```python
from build123d import *

# Parameters (mm, degrees)
SKETCH_3_R      = 2.25
EXTRUDE_1_DEPTH = 11
SKETCH_4_R      = 0.4
FILLET_1_R      = 0.5


with BuildPart() as part:
    # Эскиз3 → Вытянуть1 (new body)
    with BuildSketch(Plane(origin=(2.5, 0, 0), x_dir=(0, 0, -1), z_dir=(1, 0, 0))):
        with Locations((-2.25, 0)):
            Circle(SKETCH_3_R)
    extrude(amount=EXTRUDE_1_DEPTH)

    # По траектории1: sweep along a path in Эскиз5
    with BuildLine(Plane(origin=(0, 0, 0), x_dir=(1, 0, 0), z_dir=(0, 1, 0))) as sweep_1_path:
        Line((0, 5.25), (0, -0.25))
        ThreePointArc((0, -0.25), (0.585786438, -1.664213562), (2, -2.25))
        Line((2, -2.25), (2.965757317, -2.25))
        Line((2.965757317, -2.25), (14, -2.25))
        ThreePointArc((14, -2.25), (15.414213562, -1.664213562), (16, -0.25))
        Line((16, -0.25), (16, 5.25))
    # Эскиз4 → По траектории1 (sweep)
    with BuildSketch(Plane.XY.offset(-5.25)):
        Circle(SKETCH_4_R)
    sweep(path=sweep_1_path.line)

    # Скругление1
    fillet_1_edges = [part.edges().sort_by_distance(p)[0] for p in [
        (2.5, 0, 4.5),
        (13.5, 0, 4.5),
    ]]
    fillet(fillet_1_edges, radius=FILLET_1_R)


solid = part.part
```
The listing builds one solid part. Answer for the finished solid, in the listing's coordinates (mm). Give positions to 0.01 mm unless a question says otherwise; leave off trailing zeros. Order: outer loops, then holes, each group sorted by start corner. A loop starts at its lowest first (then second) coordinate and runs counter-clockwise, first axis right, second up.
1) Find section A-A on y = 0. Write down the section's boundary in (x, z).
Reported:
outline: (-0.4, -5.25) - (0.4, -5.25) - (0.4, 0.25) arc R1.6 cw to (2, 1.85) - (2.5, 1.85) - (2.5, 0.5) arc R0.5 ccw to (3, 0) - (13, 0) arc R0.5 ccw to (13.5, 0.5) - (13.5, 1.85) - (14, 1.85) arc R1.6 cw to (15.6, 0.25) - (15.6, -5.25) - (16.4, -5.25) - (16.4, 0.25) arc R2.4 ccw to (14, 2.65) - (13.5, 2.65) - (13.5, 4) arc R0.5 ccw to (13, 4.5) - (3, 4.5) arc R0.5 ccw to (2.5, 4) - (2.5, 2.65) - (2, 2.65) arc R2.4 ccw to (-0.4, 0.25) - close
2) Given P1, Ø1, axis at x = 4.5, z = 0, coming from the -Y side; P2, Ø1, axis at y = 0, z = 1.5, coming from the -X side; P3, Ø4, axis at x = 12.5, z = 0, coming from the -Y side, each flat-ended and moving along its own axis, determine where each tip first touches the part or whether it passes through.
Reported:
P1: stops at y = -1.41
P2: stops at x = -0.28
P3: stops at y = -2.24
3) Find section D-D on z = 1.5. Give the number of separate pieces and of enclosed holes in the cut face, then the cut area to 3 significant figures.
Reported:
separate pieces: 3
enclosed holes: 0
area: 47.8 mm2
4) Consider line 1 along X through (y, z) = (-1.8, 2); line 2 along Z through (x, y) = (3, -0.05); line 3 along X through (y, z) = (0.15, 1.5). Determine where each line is inside the solid, lowest interval first.
Reported:
line 1: x = 2.5 to 13.5
line 2: z = 0 to 4.5
line 3: x = -0.01 to 0.96, 2.5 to 13.5, 15.04 to 16.01
5) Find section C-C on x = 7.5. Write down the section's boundary in (y, z).
Reported:
outline: circle Ø4.5 at (0, 2.25)
6) Find section B-B on z = -0.25. Write down the section's boundary in (x, y).
Reported:
outline: circle Ø0.8 at (0, 0); circle Ø0.8 at (16, 0)
